Work out the finished part from the listing and answer in its coordinate system (mm). Face numbers are marked on the shaded views. Give positions to 0.01 mm unless a question says otherwise; leave off trailing zeros. Write each loop counter-clockwise with the first axis right and the second up, starting at its lowest first coordinate (ties: lowest second). Pieces come first, ordered by that corner, then holes.
1) Find section C-C (y = 16). Determine the outline of the cut face in (x, z), plus the area to 3 significant figures.
2) Straight lines are drawn through the part: probe 1 along Y at (x, z) = (25, 1.15); probe 2 along Y at (x, z) = (2.5, 1.45); probe 3 along Y at (x, z) = (22, 1.2). For each, find the intervals that lie inside material, in ascending order.
3) Find section A-A (y = 0). Determine the outline of the cut face in (x, z), plus the area to 3 significant figures.
4) Given pin 1 Ø1 at (y, z) = (0.5, 0.5) entering from -X; pin 2 Ø1.1 at (x, z) = (1, 1.5) entering from -Y, each flat-ended and moving along its own axis, determine where each tip first touches the part or whether it passes through.
5) Determine the mould class of the marked faces 1 and 2 for opening direction X: pulls with the +X half, pulls with the -X half, needs draft (parallel to the pull), parting line crosses it, or undercut.
```python
from build123d import *

# Parameters (mm, degrees)
F1_DEPTH = 2
F3_DEPTH = 1


with BuildPart() as f1:
    # F0 (on Top) → F1 (new body)
    with BuildSketch(Plane.XY):
        with BuildLine():
            Line((12.5, -27), (40.5, -27))
            ThreePointArc((40.5, -27), (41.914214, -26.414214), (42.5, -25))
            Line((42.5, -25), (42.5, 25))
            ThreePointArc((42.5, 25), (41.914214, 26.414214), (40.5, 27))
            Line((40.5, 27), (12.5, 27))
            ThreePointArc((12.5, 27), (11.914214, 25.585786), (10.5, 25))
            Line((10.5, 25), (-10.5, 25))
            ThreePointArc((-10.5, 25), (-11.914214, 25.585786), (-12.5, 27))
            Line((-12.5, 27), (-40.5, 27))
            ThreePointArc((-40.5, 27), (-41.914214, 26.414214), (-42.5, 25))
            Line((-42.5, 25), (-42.5, 15))
            ThreePointArc((-42.5, 15), (-27.5, 0), (-42.5, -15))
            Line((-42.5, -15), (-42.5, -25))
            ThreePointArc((-42.5, -25), (-41.914214, -26.414214), (-40.5, -27))
            Line((-40.5, -27), (-12.5, -27))
            ThreePointArc((-12.5, -27), (-11.914214, -25.585786), (-10.5, -25))
            Line((-10.5, -25), (10.5, -25))
            ThreePointArc((10.5, -25), (11.914213, -25.585787), (12.5, -27))
        make_face()
        with BuildLine():
            Line((30.5, 11), (30.5, 0))
            Line((30.5, 0), (30.5, -11))
            ThreePointArc((30.5, -11), (30.207107, -11.707107), (29.5, -12))
            Line((29.5, -12), (24.350781, -12))
            ThreePointArc((24.350781, -12), (23.567891, -11.840403), (22.909948, -11.387083))
            Line((22.909948, -11.387083), (19.059167, -7.387083))
            ThreePointArc((19.059167, -7.387083), (18.645052, -6.747775), (18.5, -6))
            Line((18.5, -6), (18.5, 0))
            Line((18.5, 0), (18.5, 6))
            ThreePointArc((18.5, 6), (18.645052, 6.747775), (19.059167, 7.387083))
            Line((19.059167, 7.387083), (22.909948, 11.387083))
            ThreePointArc((22.909948, 11.387083), (23.567891, 11.840403), (24.350781, 12))
            Line((24.350781, 12), (29.5, 12))
            ThreePointArc((29.5, 12), (30.207107, 11.707107), (30.5, 11))
        make_face(mode=Mode.SUBTRACT)
    extrude(amount=F1_DEPTH)

    # F2 (on face) → F3 (cut)
    with BuildSketch(Plane.XY.offset(2)):
        with BuildLine():
            Line((-10.5, -20), (10.5, -20))
            ThreePointArc((10.5, -20), (13.145751, -20.519259), (15.398979, -22))
            Line((15.398979, -22), (37.5, -22))
            Line((37.5, -22), (37.5, 22))
            Line((37.5, 22), (15.398979, 22))
            ThreePointArc((15.398979, 22), (13.145751, 20.519259), (10.5, 20))
            Line((10.5, 20), (-10.5, 20))
            ThreePointArc((-10.5, 20), (-13.145751, 20.519259), (-15.398979, 22))
            Line((-15.398979, 22), (-37.5, 22))
            Line((-37.5, 22), (-37.5, 19.364917))
            ThreePointArc((-37.5, 19.364917), (-22.5, 0), (-37.5, -19.364917))
            Line((-37.5, -19.364917), (-37.5, -22))
            Line((-37.5, -22), (-15.398979, -22))
            ThreePointArc((-15.398979, -22), (-13.145751, -20.519259), (-10.5, -20))
        make_face()
        with BuildLine():
            ThreePointArc((29.5, 15), (32.328427, 13.828427), (33.5, 11))
            Line((33.5, 11), (33.5, -11))
            ThreePointArc((33.5, -11), (32.328427, -13.828427), (29.5, -15))
            Line((29.5, -15), (24.350781, -15))
            ThreePointArc((24.350781, -15), (22.393556, -14.601008), (20.748698, -13.467708))
            Line((20.748698, -13.467708), (16.897917, -9.467708))
            ThreePointArc((16.897917, -9.467708), (15.862629, -7.869437), (15.5, -6))
            Line((15.5, -6), (15.5, 6))
            ThreePointArc((15.5, 6), (15.862629, 7.869437), (16.897917, 9.467708))
            Line((16.897917, 9.467708), (20.748698, 13.467708))
            ThreePointArc((20.748698, 13.467708), (22.393556, 14.601008), (24.350781, 15))
            Line((24.350781, 15), (29.5, 15))
        make_face(mode=Mode.SUBTRACT)
    extrude(amount=-F3_DEPTH, mode=Mode.SUBTRACT)


solid = f1.part
```
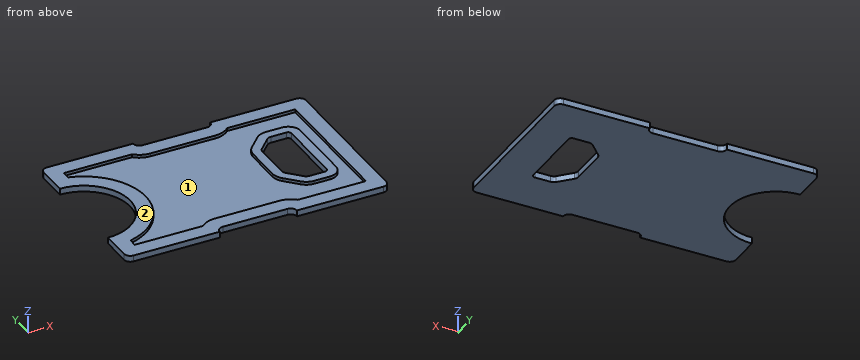
Results:
1. outline: (-42.5, 0) - (42.5, 0) - (42.5, 2) - (37.5, 2) - (37.5, 1) - (-30.5, 1) - (-30.5, 2) - (-42.5, 2) - close
1. area: 102 mm2
2. probe 1: y = -27 to -22, -15 to -12, 12 to 15, 22 to 27
2. probe 2: y = -25 to -20, 20 to 25
2. probe 3: y = -27 to -22, -14.41 to -10.44, 10.44 to 14.41, 22 to 27
3. outline: (-27.5, 0) - (18.5, 0) - (18.5, 2) - (15.5, 2) - (15.5, 1) - (-22.5, 1) - (-22.5, 2) - (-27.5, 2) - close; (30.5, 0) - (42.5, 0) - (42.5, 2) - (37.5, 2) - (37.5, 1) - (33.5, 1) - (33.5, 2) - (30.5, 2) - close
3. area: 74.0 mm2
4. pin 1: stops at x = -27.53
4. pin 2: stops at y = -25
5. face 1: undercut
5. face 2: needs draft
